Check sheet for the modelled part. Datum: model origin and axes. Units: mm. Round coordinates to 2 decimals unless told otherwise and drop trailing zeros. Write each loop counter-clockwise with the first axis right and the second up, starting at its lowest first coordinate (ties: lowest second). Pieces come first, ordered by that corner, then holes. Notation, with made-up numbers: (50, 56) -> (106, 56) arc R16 cw to (106, 85) -> close; hole circle Ø2 at (-23.75, 1). An arc over 180 degrees is marked (long way). One line per item, written item: value. Start each with the question number.
```python
from build123d import *

# Parameters (mm, degrees)
F0_R     = 10
F1_DEPTH = 20
F2_W     = 32
F2_H     = 21
F3_DEPTH = 4
F4_R     = 5
F5_DEPTH = 25
F6_R     = 5


with BuildPart() as f1:
    # F0 (on Top) → F1 (new body)
    with BuildSketch(Plane.XY):
        Circle(F0_R)
    extrude(amount=F1_DEPTH)

    # F2 (on face) → F3 (join)
    with BuildSketch(Plane.XY.offset(20)):
        Rectangle(F2_W, F2_H)
    extrude(amount=F3_DEPTH)

    # F4 (on face) → F5 (cut)
    with BuildSketch(Plane.XY.offset(24)):
        Circle(F4_R)
    extrude(amount=-F5_DEPTH, mode=Mode.SUBTRACT)

    # F6
    f6_edges = [f1.edges().sort_by_distance(p)[0] for p in [
        (16, 10.5, 22),
        (-16, 10.5, 22),
        (-16, -10.5, 22),
        (16, -10.5, 22),
    ]]
    fillet(f6_edges, radius=F6_R)


solid = f1.part
```
1. Release check for a two-part mould opening along Y. For faces 1 (the face through (-2.17, -9.76, 9.86)), 2 (the face through (-5, -2, 0)), 3 (the face through (0, -10.5, 22)), 4 (the face through (-1.08, -4.88, 12.17)) record: +Y half, -Y half, draft (parallel to the pull), parting line (faces both ways), or undercut.
2. Cross-section at D-D (x = 8). Record the cut outline in (y, z).
3. Cross-section at B-B (y = 1). Record the cut outline in (x, z), plus the area to 3 significant figures.
4. Depth check by flat-ended pin: pin 1 Ø8 at (y, z) = (7.5, 13) entering from -X; pin 2 Ø12 at (x, z) = (-8.5, 10.5) entering from -Y; pin 3 Ø3 at (y, z) = (6.5, 10) entering from -X. Enter the tip coordinate at first touch or a pass-through.
5. Cross-section at A-A (x = 0). Record the cut outline in (y, z), plus the area to 3 significant figures.
6. Material ranges on probe 1 along Y at (x, z) = (0, 18); probe 2 along Z at (x, y) = (10, -5.25); probe 3 along X at (y, z) = (0.5, 11.5), recorded low to high.
7. Cross-section at C-C (z = 9.5). Record the cut outline in (x, y), plus the area to 3 significant figures.
Working result:
1. face 1: parting line
1. face 2: draft
1. face 3: -Y half
1. face 4: undercut
2. outline: (-10.5, 20) -> (-6, 20) -> (-6, 0) -> (6, 0) -> (6, 20) -> (10.5, 20) -> (10.5, 24) -> (-10.5, 24) -> close
3. outline: (-16, 20) -> (-9.95, 20) -> (-9.95, 0) -> (-4.9, 0) -> (-4.9, 24) -> (-16, 24) -> close; (4.9, 0) -> (9.95, 0) -> (9.95, 20) -> (16, 20) -> (16, 24) -> (4.9, 24) -> close
3. area: 291 mm^2
4. pin 1: stops at x = -9.37
4. pin 2: stops at y = -9.68
4. pin 3: stops at x = -8.66
5. outline: (-10.5, 20) -> (-10, 20) -> (-10, 0) -> (-5, 0) -> (-5, 24) -> (-10.5, 24) -> close; (5, 0) -> (10, 0) -> (10, 20) -> (10.5, 20) -> (10.5, 24) -> (5, 24) -> close
5. area: 244 mm^2
6. probe 1: y = -10 to -5, 5 to 10
6. probe 2: z = 20 to 24
6. probe 3: x = -9.99 to -4.97, 4.97 to 9.99
7. outline: circle Ø20 at (0, 0); hole circle Ø10 at (0, 0)
7. area: 236 mm^2
